Input: part model. Units: mm. Frame: model coordinates. Face numbers are marked on the shaded views. A direction names the side the tool comes from. Coordinates: 2 decimals unless noted, no trailing zeros. Loops run counter-clockwise (first coordinate to the right, second up) from the corner with the lowest first, then second, coordinate; pieces in that order, holes last.
(1) Mould query, pull axis Y, two halves, no side actions, for the marked faces 1, 2 and 3. Classes: released by +Y, released by -Y, zero draft, split by the parting line, or undercut.
(2) Line query: L1, parallel to X at y = 0, z = 36.1; L2, parallel to Z at x = -1, y = -2. Output: solid intervals per line, ascending.
(3) Contact query for flat-ended pins moving along their axis: P1, Ø6, axis at y = 4.5, z = 11, coming from the +X side; P2, Ø6, axis at x = 0, y = 3, coming from the -Z side; P3, Ø10, axis at x = -2, y = 3, coming from the +Z side; P4, Ø6, axis at x = 3, z = 27.5, coming from the +Y side. Output: stop coordinate, or through.
(4) Section C-C, the plane z = 26. Return loops of the section in (x, y), then the cut area to 3 significant figures.
(5) Set-up query: the marked faces 4 and 5. Return all of +Z, -Z, +X, -X, +Y, -Y with unobstructed straight access to the full face (end or side cutting, diameter ignored); none if empty.
```python
from build123d import *

# Parameters (mm, degrees)
F0_R     = 2
F1_DEPTH = 35
F2_R     = 10
F3_DEPTH = 3


with BuildPart() as f1:
    # F0 (on Top) → F1 (new body)
    with BuildSketch(Plane.XY):
        Circle(F0_R)
    extrude(amount=F1_DEPTH)

    # F2 (on face) → F3 (join)
    with BuildSketch(Plane.XY.offset(35)):
        Circle(F2_R)
    extrude(amount=F3_DEPTH)

    # F5 (on Right) → F6 (revolve)
    with BuildSketch(Plane.YZ):
        Polygon((0, 31.303294), (0, 35.309382), (-10.035225, 35.309382), (-4.777231, 27.397355), (0, 27.247125), align=None)
    revolve(axis=Axis((0, 0, 31.278254), (0, 0, -1)))

    # F7 (on Front) → F8 (revolve, cut)
    with BuildSketch(Plane.XZ):
        Polygon((9.262677, 40.559426), (0, 38.892001), (0, 35.140295), (9.262677, 35.140295), align=None)
    revolve(axis=Axis((0, 0, 37.016148), (0, 0, -1)), mode=Mode.SUBTRACT)


solid = f1.part
```
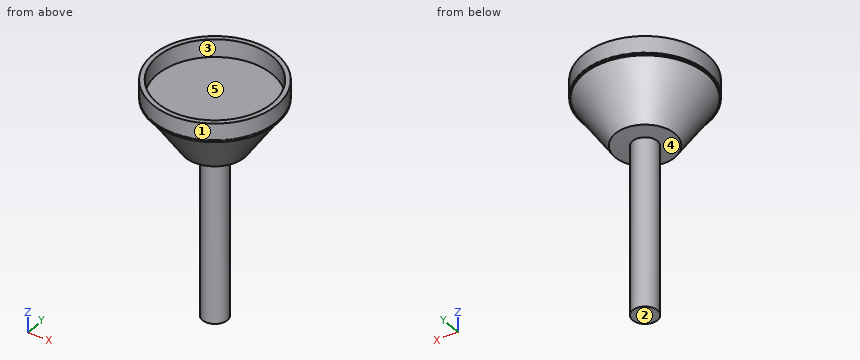
Report:
1. face 1: split by the parting line
1. face 2: zero draft
1. face 3: undercut
2. L1: x = -10 to -9.26, 9.26 to 10
2. L2: z = 27.32 to 35.14
3. P1: stops at x = 1.32
3. P2: stops at z = 0
3. P3: stops at z = 35.14
3. P4: stops at y = 6.43
4. outline: circle Ø4 at (0, 0)
4. area: 12.6 mm2
5. face 4: -Z
5. face 5: +Z
